Source: CAD feature listing. Evaluate the final solid. Frame: model axes, mm. Coordinates: 2 decimals unless noted, no trailing zeros. Write each loop counter-clockwise with the first axis right and the second up, starting at its lowest first coordinate (ties: lowest second). Pieces come first, ordered by that corner, then holes. Notation, with made-up numbers: (62, -7.75) - (101, -7.75) arc R20 cw to (101, -1.75) - close; hole circle Ø2 at (20.25, 16). An arc over 180 degrees is marked (long way). One line per question, with ' | ' between items. Start each with the question number.
Q1. Cut plane B-B, the plane y = 21.5. Return loops of the section in (x, z), plus the area to 3 significant figures.
Q2. Line query: line 1 (Y direction, x = 24.5, z = 0.9); line 2 (Y direction, x = 4, z = 0.75); line 3 (X direction, y = 42.5, z = 1.4). Output: solid intervals per line, ascending.
Q3. Cut plane D-D, the plane z = 1.3. Give the number of separate pieces and of enclosed holes in the cut face, plus the area to 3 significant figures.
Q4. Contact query for a flat-ended pin moving along its axis: P1, Ø4.5, axis at x = 24.5, y = 42.54, coming from the +Z side. Output: stop coordinate, or through.
Q5. Cut plane C-C, the plane x = 124. Return loops of the section in (y, z).
Q6. Cut plane A-A, the plane x = 69.5. Return loops of the section in (y, z).
```python
from build123d import *

# Parameters (mm, degrees)
SKETCH1_W           = 139
SKETCH1_H           = 52
SKETCH1_R           = 1.6
SKETCH1_R_2         = 3.75
SKETCH1_W_2         = 3.2
SKETCH1_H_2         = 1.9
SKETCH1_W_3         = 2.2
SKETCH1_H_3         = 1.1
BOSS_EXTRUDE1_DEPTH = 3


with BuildPart() as part:
    # Sketch1 → Boss-Extrude1 (new body)
    with BuildSketch(Plane.XY):
        with Locations((69.5, 26)):
            Rectangle(SKETCH1_W, SKETCH1_H)
        with Locations((4, 35.5)):
            Circle(SKETCH1_R, mode=Mode.SUBTRACT)
        with Locations((135, 35.5)):
            Circle(SKETCH1_R, mode=Mode.SUBTRACT)
        with Locations((135, 13.5)):
            Circle(SKETCH1_R, mode=Mode.SUBTRACT)
        with Locations((4, 13.5)):
            Circle(SKETCH1_R, mode=Mode.SUBTRACT)
        with Locations((14.309088021, 21.5)):
            Circle(SKETCH1_R, mode=Mode.SUBTRACT)
        with Locations((124, 28.19419762)):
            Circle(SKETCH1_R, mode=Mode.SUBTRACT)
        with Locations((69.5, 15.301613352)):
            Circle(SKETCH1_R_2, mode=Mode.SUBTRACT)
        with Locations((24.5, 42.541519479)):
            Circle(SKETCH1_R_2, mode=Mode.SUBTRACT)
        with Locations((54.5, 42.541519479)):
            Circle(SKETCH1_R_2, mode=Mode.SUBTRACT)
        with Locations((84.5, 42.541519479)):
            Circle(SKETCH1_R_2, mode=Mode.SUBTRACT)
        with Locations((114.5, 42.541519479)):
            Circle(SKETCH1_R_2, mode=Mode.SUBTRACT)
        with Locations((69.5, 7.601613352)):
            Rectangle(SKETCH1_W_2, SKETCH1_H_2, mode=Mode.SUBTRACT)
        with Locations((24.5, 36.291519479)):
            Rectangle(SKETCH1_W_3, SKETCH1_H_3, mode=Mode.SUBTRACT)
        with BuildLine():
            Line((100.339676821, 12.351613352), (104.466418878, 12.351613352))
            ThreePointArc((104.466418878, 12.351613352), (106.003047849, 15.301613352), (104.466418878, 18.251613352))
            Line((104.466418878, 18.251613352), (100.339676821, 18.251613352))
            ThreePointArc((100.339676821, 18.251613352), (98.803047849, 15.301613352), (100.339676821, 12.351613352))
        make_face(mode=Mode.SUBTRACT)
        with BuildLine():
            Line((29.767863143, 12.351613352), (33.894605199, 12.351613352))
            ThreePointArc((33.894605199, 12.351613352), (35.431234171, 15.301613352), (33.894605199, 18.251613352))
            Line((33.894605199, 18.251613352), (29.767863143, 18.251613352))
            ThreePointArc((29.767863143, 18.251613352), (28.231234171, 15.301613352), (29.767863143, 12.351613352))
        make_face(mode=Mode.SUBTRACT)
        with Locations((54.5, 36.291519479)):
            Rectangle(SKETCH1_W_3, SKETCH1_H_3, mode=Mode.SUBTRACT)
        with Locations((84.5, 36.291519479)):
            Rectangle(SKETCH1_W_3, SKETCH1_H_3, mode=Mode.SUBTRACT)
        with Locations((114.5, 36.291519479)):
            Rectangle(SKETCH1_W_3, SKETCH1_H_3, mode=Mode.SUBTRACT)
    extrude(amount=BOSS_EXTRUDE1_DEPTH)


solid = part.part
```
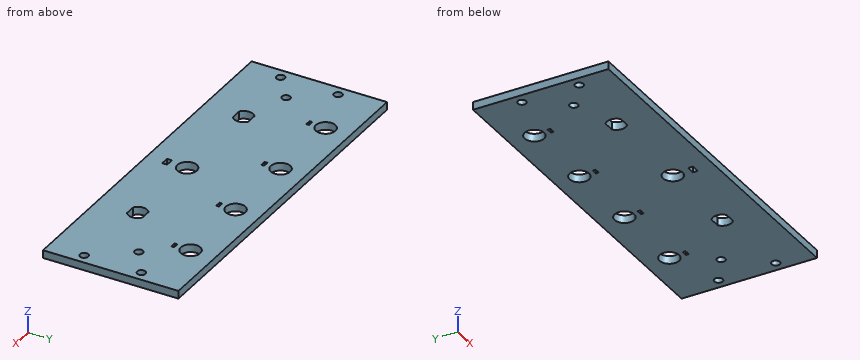
Reply:
1) outline: (0, 0) - (12.71, 0) - (12.71, 3) - (0, 3) - close; (15.91, 0) - (139, 0) - (139, 3) - (15.91, 3) - close | area: 407 mm^2
2) line 1: y = 0 to 35.74, 36.84 to 38.79, 46.29 to 52 | line 2: y = 0 to 11.9, 15.1 to 33.9, 37.1 to 52 | line 3: x = 0 to 20.75, 28.25 to 50.75, 58.25 to 80.75, 88.25 to 110.75, 118.25 to 139
3) separate pieces: 1 | enclosed holes: 18 | area: 6,870 mm^2
4) P1: passes through
5) outline: (0, 0) - (26.59, 0) - (26.59, 3) - (0, 3) - close; (29.79, 0) - (52, 0) - (52, 3) - (29.79, 3) - close
6) outline: (0, 0) - (6.65, 0) - (6.65, 3) - (0, 3) - close; (8.55, 0) - (11.55, 0) - (11.55, 3) - (8.55, 3) - close; (19.05, 0) - (52, 0) - (52, 3) - (19.05, 3) - close
